Geometry: final body of the model. Coordinates: model frame, mm. Face numbers are marked on the shaded views. A direction names the side the tool comes from. Give positions to 0.01 mm unless a question says otherwise; leave off trailing zeros. Write each loop counter-clockwise with the first axis right and the second up, starting at its lowest first coordinate (ties: lowest second). Pieces come first, ordered by that corner, then holes. Notation, with made-up numbers: M 12,45.25 L 60,45.25 A23 ccw 60,67.25 Z; hole C -27,-23 d4. An arc over 180 degrees is marked long. Answer as a JSON object with one key per item and string values.
from build123d import *

# Parameters (mm, degrees)
SKETCH_1_W          = 80
SKETCH_1_H          = 40
EXTRUDE_1_DEPTH     = 30
SKETCH_2_W          = 40
SKETCH_2_H          = 13.147576883
CUT_EXTRUDE_1_DEPTH = 65.031242374
CUT_EXTRUDE_2_DEPTH = 10
SKETCH_5_R          = 15
EXTRUDE_2_DEPTH     = 10
EXTRUDE_START       = 30
SKETCH_6_R          = 20
SKETCH_6_R_2        = 15
EXTRUDE_3_DEPTH     = 30


with BuildPart() as part:
    # 草圖1 → 填料-伸長1 (new body)
    with BuildSketch(Plane.XY):
        Rectangle(SKETCH_1_W, SKETCH_1_H)
    extrude(amount=EXTRUDE_1_DEPTH)

    # 草圖2 → 除料-伸長1 (cut, through all)
    with BuildSketch(Plane.XZ.offset(20)):
        with Locations((0, 3.426211558)):
            Rectangle(SKETCH_2_W, SKETCH_2_H)
    extrude(amount=-CUT_EXTRUDE_1_DEPTH, mode=Mode.SUBTRACT)

    # 草圖3 → 除料-伸長2 (cut)
    with BuildSketch(Plane.XY.offset(30)):
        with BuildLine():
            Line((15, -10), (-5, -10))
            ThreePointArc((-5, -10), (-15, 0), (-5, 10))
            Line((-5, 10), (15, 10))
            ThreePointArc((15, 10), (25, 0), (15, -10))
        make_face()
    extrude(amount=-CUT_EXTRUDE_2_DEPTH, mode=Mode.SUBTRACT)

    # 草圖5 → 填料-伸長2 (add)
    with BuildSketch(Plane.ZY.offset(40)):
        with BuildLine():
            Line((30, -20), (60, -20))
            ThreePointArc((60, -20), (80, 0), (60, 20))
            Line((60, 20), (30, 20))
            Line((30, 20), (30, -20))
        make_face()
        with Locations((60, 0)):
            Circle(SKETCH_5_R, mode=Mode.SUBTRACT)
    extrude(amount=-EXTRUDE_2_DEPTH)

    # 草圖6 → 填料-伸長3 (add)
    with BuildSketch(Plane.ZY.offset(40).offset(EXTRUDE_START)):
        with Locations((60, 0)):
            Circle(SKETCH_6_R)
        with Locations((60, 0)):
            Circle(SKETCH_6_R_2, mode=Mode.SUBTRACT)
    extrude(amount=-EXTRUDE_3_DEPTH)


solid = part.part
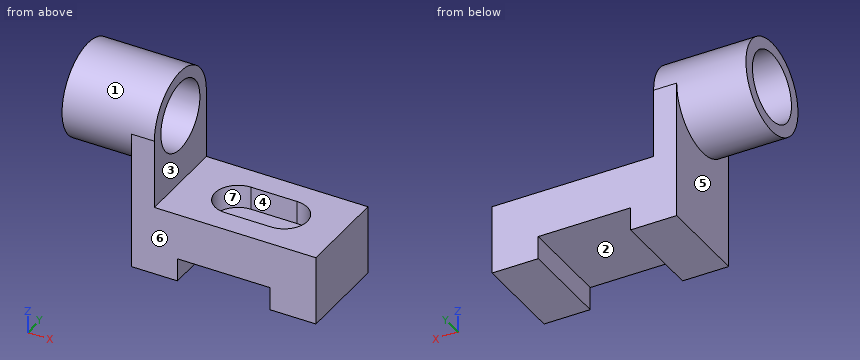
1) Set-up query: the marked faces 1, 2 and 3. Return all of +Z, -Z, +X, -X, +Y, -Y with unobstructed straight access to the full face (end or side cutting, diameter ignored); none if empty.
Geometry check:
{"face 1": "-X", "face 2": "-Z, +Y, -Y", "face 3": "+Z, +X, +Y, -Y"}
2) Cut plane C-C on x = -61.5. Return loops of the section in (y, z).
Geometry check:
{"outline": "C 0,60 d40; hole C 0,60 d30"}
3) Contact query for flat-ended pins moving along their axis: P1, Ø5, axis at y = -15.5, z = 59.5, coming from the +X side; P2, Ø6, axis at x = -4.5, y = -1.5, coming from the +Z side; P3, Ø8, axis at y = -1.5, z = 4.5, coming from the -X side. Output: stop coordinate, or through.
Geometry check:
{"P1": "stops at x = -30", "P2": "stops at z = 20", "P3": "stops at x = -40"}
4) Line query: line 1 (Y direction, x = -56, z = 60); line 2 (Y direction, x = 1.5, z = 23); line 3 (X direction, y = -2, z = 4). Output: solid intervals per line, ascending. Write a range as from..to.
Geometry check:
{"line 1": "y = -20..-15, 15..20", "line 2": "y = -20..-10, 10..20", "line 3": "x = -40..-20, 20..40"}
5) Cut plane D-D on z = 16. Return loops of the section in (x, y), and give its area (3 significant figures).
Geometry check:
{"outline": "M -40,-20 L 40,-20 L 40,20 L -40,20 Z", "area": "3,200 mm2"}
6) Pull-direction query (Y, two-part tool) for the marked faces 4, 5, 6 and 7; classes: pulls with the +Y half, pulls with the -Y half, needs draft (parallel to the pull), parting line crosses it, or undercut.
Geometry check:
{"face 4": "undercut", "face 5": "needs draft", "face 6": "pulls with the -Y half", "face 7": "undercut"}
7) Cut plane B-B on y = 16.5. Return loops of the section in (x, z), and give its area (3 significant figures).
Geometry check:
{"outline": "M -70,48.7 L -40,48.7 L -40,0 L -20,0 L -20,10 L 20,10 L 20,0 L 40,0 L 40,30 L -30,30 L -30,71.3 L -70,71.3 Z", "area": "3,090 mm2"}
8) Cut plane A-A on y = 11.5. Return loops of the section in (x, z).
Geometry check:
{"outline": "M -70,43.64 L -40,43.64 L -40,0 L -20,0 L -20,10 L 20,10 L 20,0 L 40,0 L 40,30 L -30,30 L -30,50.37 L -70,50.37 Z; M -70,69.63 L -30,69.63 L -30,76.36 L -70,76.36 Z"}
